from build123d import *

# Parameters (mm, degrees)
SKETCH1_R           = 6
BASE_EXTRUDE_DEPTH  = 180
SKETCH2_R           = 6.05
BOSS_EXTRUDE1_DEPTH = 10
BOSS_EXTRUDE2_START = 210
SKETCH3_R           = 6
BOSS_EXTRUDE2_DEPTH = 210
SKETCH4_R           = 45
BOSS_EXTRUDE3_DEPTH = 8
SCALE1_SCALE        = 4


with BuildPart() as part:
    # Sketch1 → Base-Extrude (new body)
    with BuildSketch(Plane(origin=(0, 0, 0), x_dir=(1, 0, 0), z_dir=(0, 1, 0))):
        with Locations(Location((0, 0, 0), (0, 0, 90))):
            Circle(SKETCH1_R)
    extrude(amount=BASE_EXTRUDE_DEPTH)

    # Sketch2 → Boss-Extrude1 (add)
    with BuildSketch(Plane.XZ):
        with Locations(Location((0, 0, 0), (0, 0, 270))):
            Circle(SKETCH2_R)
    extrude(amount=BOSS_EXTRUDE1_DEPTH)

    # Sketch3 → Boss-Extrude2 (add)
    with BuildSketch(Plane.XZ.offset(10).offset(BOSS_EXTRUDE2_START)):
        with Locations(Location((0, 0, 0), (0, 0, 270))):
            Circle(SKETCH3_R)
    extrude(amount=-BOSS_EXTRUDE2_DEPTH)

    # Sketch4 → Boss-Extrude3 (add)
    with BuildSketch(Plane.XZ.offset(220)):
        with Locations(Location((0, 0, 0), (0, 0, 270))):
            Circle(SKETCH4_R)
    extrude(amount=BOSS_EXTRUDE3_DEPTH)

    # Sketch5 → Boss-Revolve-Thin1 (revolve)
    with BuildSketch(Plane.XY, mode=Mode.PRIVATE) as boss_revolve_thin1_sk:
        with BuildLine():
            Line((0, 179.958378868), (8.34246908, 179.958378868))
            ThreePointArc((8.34246908, 179.958378868), (38.657452483, 187.592823497), (61.740544461, 208.674897119))
            Line((61.740544461, 208.674897119), (62.574826169, 208.123558718))
            ThreePointArc((62.574826169, 208.123558718), (39.131088208, 186.712102655), (8.34246908, 178.958378868))
            Line((8.34246908, 178.958378868), (0, 178.958378868))
            Line((0, 178.958378868), (0, 179.958378868))
        make_face()
    revolve(boss_revolve_thin1_sk.sketch.rotate(Axis((0, 208.674897119, 0), (0, -1, 0)), 90), axis=Axis((0, 208.674897119, 0), (0, -1, 0)))


with BuildPart() as part_1:
    # Scale1: scaled about (0, -84.253032849, 0)
    add(part.part.scale(SCALE1_SCALE).moved(Location((0, 252.759098547, 0))))


solid = part_1.part
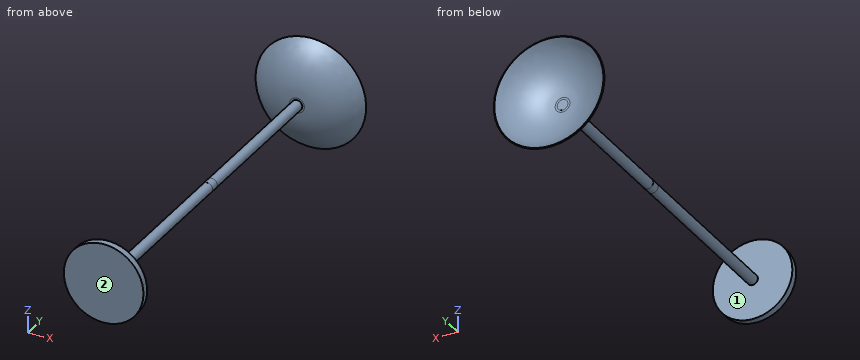
CAD build for the part. Positions are in the model's coordinates, mm. Face numbers are marked on the shaded views. Round coordinates to 2 decimals unless told otherwise and drop trailing zeros. Order: outer loops, then holes, each group sorted by start corner. A loop starts at its lowest first (then second) coordinate and runs counter-clockwise, first axis right, second up. Notation, with made-up numbers: (-13, -29) -> (-5, -29) arc R27 cw to (-5, -7) -> close; hole circle Ø5 at (75.5, -29). An arc over 180 degrees is marked (long way). Write item = value, one per line. Start each with the question number.
(1) Cut at A-A, the plane y = 538.5. List the corners of the cut face in (x, z), then the cut area to 3 significant figures.
(2) Pull direction Y, two halves, no side cores. Call the marked faces 1 and 2: released by +Y, released by -Y, zero draft, split by the parting line, or undercut.
(3) Probe line 1 (Y direction, x = 113.5, z = 96); line 2 (Z direction, x = -3, y = 514); line 3 (Y direction, x = -21.5, z = -5). List the from-to ranges inside material, lowest first. Write a range as [from, to].
(4) Pin check, flat tips, straight feed: P1, Ø4, axis at y = 60.5, z = 12, coming from the -X side; P2, Ø1.5, axis at x = -107, z = -169.5, coming from the +Y side; P3, Ø1, axis at x = 21.5, z = -75.5, coming from the +Y side. Stop position of each tip, or through.
Model answer:
q1.outline = circle Ø48 at (0, 0)
q1.area = 1,810 mm2
q2.face_1 = undercut
q2.face_2 = released by -Y
q3.line_1 = [-659.24, -627.24], [995.55, 1000.02]
q3.line_2 = [-23.81, 23.81]
q3.line_3 = [-659.24, 972.76]
q4.P1 = -21.82
q4.P2 = 1035.27
q4.P3 = 976.69
